from build123d import *

# Parameters (mm, degrees)
F0_R     = 8.5
F1_DEPTH = 4
F2_R     = 5
F3_DEPTH = 100
F8_R     = 1.5
F9_DEPTH = 109.5


with BuildPart() as f1:
    # F0 (on Top) → F1 (new body)
    with BuildSketch(Plane.XY):
        Circle(F0_R)
    extrude(amount=F1_DEPTH)

    # F2 (on Top) → F3 (join)
    with BuildSketch(Plane.XY):
        Circle(F2_R)
    extrude(amount=F3_DEPTH)

    # F4 (on Right) → F5 (revolve)
    with BuildSketch(Plane.YZ):
        with BuildLine():
            Line((3, 102), (0, 102))
            Line((0, 102), (0, 100))
            Line((0, 100), (5, 100))
            ThreePointArc((5, 100), (3.585786, 100.585786), (3, 102))
        make_face()
    revolve(axis=Axis((0, 0, 101), (0, 0, -1)))

    # F6 (on Right) → F7 (revolve)
    with BuildSketch(Plane.YZ):
        with BuildLine():
            Line((0, 105), (0, 102))
            Line((0, 102), (3, 102))
            ThreePointArc((3, 102), (2.12132, 104.12132), (0, 105))
        make_face()
    revolve(axis=Axis((0, 0, 103.5), (0, 0, 1)))

    # F8 (on Top) → F9 (cut)
    with BuildSketch(Plane.XY):
        Circle(F8_R)
    extrude(amount=F9_DEPTH, mode=Mode.SUBTRACT)


solid = f1.part
Input: part model. Units: mm. Frame: model coordinates. A direction names the side the tool comes from. Coordinates: 2 decimals unless noted, no trailing zeros. Write each loop counter-clockwise with the first axis right and the second up, starting at its lowest first coordinate (ties: lowest second). Pieces come first, ordered by that corner, then holes. Notation, with made-up numbers: M 31,11 L 74,11 A15 ccw 74,24 Z; hole C -18.75,-21 d7. An arc over 180 degrees is marked long. Answer as a JSON object with one key per item and string values. Group by question number.
(1) Section B-B on x = 6.5. Output: boundary loops of the cut face in (y, z).
(2) Set-up query: faces 1 (the face through (-1.08, -4.88, 51.33)), 2 (the face through (2, 0, 0)). Return all of +Z, -Z, +X, -X, +Y, -Y with unobstructed straight access to the full face (end or side cutting, diameter ignored); none if empty.
(3) Contact query for flat-ended pins moving along their axis: P1, Ø10, axis at y = -3.5, z = 33, coming from the -X side; P2, Ø8, axis at x = 1.5, z = 12, coming from the +Y side; P3, Ø2.5, axis at x = 0, y = 0, coming from the +Z side; P4, Ø2, axis at y = -2.5, z = 14.5, coming from the +X side. Output: stop coordinate, or through.
(4) Mould query, pull axis Y, two halves, no side actions, for faces 3 (the face through (4.57, 7.167, 1.972)), 4 (the face through (-1.5, 0.07, 51.57)), 5 (the face through (4, -4, 4)). Classes: pulls with the +Y half, pulls with the -Y half, needs draft (parallel to the pull), parting line crosses it, or undercut.
(5) Ray query, line 1 along X through (y, z) = (0, 45); line 2 along Z through (x, y) = (4, -5.75). Return the intervals inside material, ascending. Write a range as [from, to].
(6) Section A-A on z = 61. Output: boundary loops of the cut face in (x, y).
Result set:
{
 "1": {"outline": "M -5.48,0 L 5.48,0 L 5.48,4 L -5.48,4 Z"},
 "2": {"face 1": "+Z", "face 2": "-Z, +X, -X, +Y, -Y"},
 "3": {"P1": "stops at x = -5", "P2": "stops at y = 5", "P3": "passes through", "P4": "stops at x = 4.77"},
 "4": {"face 3": "parting line crosses it", "face 4": "undercut", "face 5": "needs draft"},
 "5": {"line 1": "x = [-5, -1.5], [1.5, 5]", "line 2": "z = [0, 4]"},
 "6": {"outline": "C 0,0 d10; hole C 0,0 d3"}
}
